Design review of the part built by this model. Coordinates are the model's own, in mm. Face numbers are marked on the shaded views. Round coordinates to 2 decimals unless told otherwise and drop trailing zeros. Write each loop counter-clockwise with the first axis right and the second up, starting at its lowest first coordinate (ties: lowest second). Pieces come first, ordered by that corner, then holes. Notation, with made-up numbers: M 52.5,18.25 L 86.5,18.25 A18 cw 86.5,28.25 Z; hole C 13,48 d8. An arc over 180 degrees is marked long. Use CSV: the item, a comma, the result in double quotes.
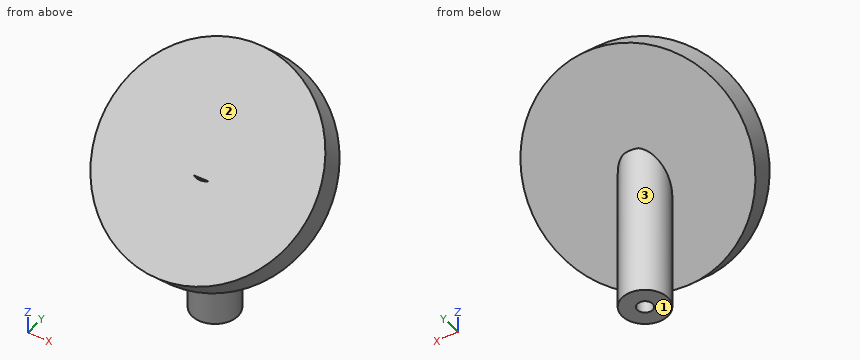
from build123d import *

# Parameters (mm, degrees)
SKETCH1_R           = 7.5
BOSS_EXTRUDE1_DEPTH = 50
SKETCH3_R           = 35
BOSS_EXTRUDE2_DEPTH = 5
SKETCH4_R           = 2.5
CUT_EXTRUDE1_DEPTH  = 5


with BuildPart() as part:
    # Sketch1 → Boss-Extrude1 (new body)
    with BuildSketch(Plane.XY):
        Circle(SKETCH1_R)
    extrude(amount=-BOSS_EXTRUDE1_DEPTH)

    # Sketch3 → Boss-Extrude2 (add, symmetric)
    with BuildSketch(Plane(origin=(0, 0, 0), x_dir=(1, 0, 0), z_dir=(0, -0.7071067811865475, 0.7071067811865477))):
        with Locations(Location((0, 0, 0), (0, 0, 270))):
            Circle(SKETCH3_R)
    extrude(amount=BOSS_EXTRUDE2_DEPTH, both=True)

    # Sketch4 → Cut-Extrude1 (cut)
    with BuildSketch(Plane(origin=(0, 0, -50), x_dir=(-1, 0, 0), z_dir=(0, 0, -1))):
        Circle(SKETCH4_R)
    extrude(amount=-CUT_EXTRUDE1_DEPTH, mode=Mode.SUBTRACT)


solid = part.part
1) Wall thickness on line 1 along Y through (x, z) = (0, -47.1); line 2 along Y through (x, z) = (0, -29.5); line 3 along Z through (x, y) = (-12, 13.5): over which ranges is each line inside the solid? List them lowest first. Write a range as [from, to].
Answers:
line 1,"[-7.5, -2.5], [2.5, 7.5]"
line 2,"[-7.5, 7.5]"
line 3,"[6.43, 20.57]"
2) Add section C-C on x = -15.5. Write out the cut boundary in (y, z).
Answers:
outline,"M -25.73,-18.65 L -18.65,-25.73 L 25.73,18.65 L 18.65,25.73 Z"
3) For pin 1 Ø3 at (x, y) = (0, 0) entering from +Z; pin 2 Ø6 at (x, z) = (23.5, -10.5) entering from -Y; pin 3 Ø4 at (x, z) = (13, -15.5) entering from -Y; pin 4 Ø4 at (x, y) = (-0.5, 1) entering from -Z, all flat-tipped, find the tip position at first contact; note any pin that passes through.
Answers:
pin 1,"z = 8.57"
pin 2,"y = -20.57"
pin 3,"y = -24.57"
pin 4,"z = -50"
4) Add section A-A on x = 0. Write out the cut boundary in (y, z), then the cut area to 3 significant figures.
Answers:
outline,"M -28.28,-21.21 L -21.21,-28.28 L -7.5,-14.57 L -7.5,-50 L -2.5,-50 L -2.5,-45 L 2.5,-45 L 2.5,-50 L 7.5,-50 L 7.5,0 L 7.07,0 L 28.28,21.21 L 21.21,28.28 L -7.07,0 L -7.5,0 L -7.5,-0.43 Z"
area,"1,320 mm²"
5) Add section D-D on x = -25.5. Write out the cut boundary in (y, z).
Answers:
outline,"M -20.49,-13.42 L -13.42,-20.49 L 20.49,13.42 L 13.42,20.49 Z"
6) The part is to be moulded in two halves that separate along Y. For the marked faces 1, 2 and 3, say which applies: released by +Y, released by -Y, zero draft, split by the parting line, or undercut.
Answers:
face 1,"zero draft"
face 2,"released by -Y"
face 3,"undercut"
7) Add section B-B on z = -31. Write out the cut boundary in (x, y), then the cut area to 3 significant figures.
Answers:
outline,"C 0,0 d15"
area,"177 mm²"
